from build123d import *

# Parameters (mm, degrees)
SKETCH1_W           = 10.414
SKETCH1_H           = 16.256
BOSS_EXTRUDE1_DEPTH = 3.175
SKETCH2_R           = 1.5875
CUT_EXTRUDE1_DEPTH  = 3.175
SKETCH3_W           = 1.3462
SKETCH3_H           = 0.635
BOSS_EXTRUDE2_DEPTH = 12.7
SKETCH4_W           = 0.2921
SKETCH4_H           = 9.398
CUT_EXTRUDE2_DEPTH  = 3.413


with BuildPart() as part:
    # Sketch1 → Boss-Extrude1 (new body)
    with BuildSketch(Plane(origin=(0, 0, 0), x_dir=(1, 0, 0), z_dir=(0, 1, 0))):
        with Locations((5.207, 8.128)):
            Rectangle(SKETCH1_W, SKETCH1_H)
    extrude(amount=BOSS_EXTRUDE1_DEPTH)

    # Sketch2 → Cut-Extrude1 (cut)
    with BuildSketch(Plane(origin=(0, 3.175, 0), x_dir=(1, 0, 0), z_dir=(0, 1, 0))):
        with Locations((5.207, 13.081)):
            Circle(SKETCH2_R)
        with Locations((10.414, 13.081)):
            Circle(SKETCH2_R)
        with Locations((0, 13.081)):
            Circle(SKETCH2_R)
    extrude(amount=-CUT_EXTRUDE1_DEPTH, mode=Mode.SUBTRACT)

    # Sketch3 → Boss-Extrude2 (add)
    with BuildSketch(Plane.XY):
        with Locations((7.747, 2.0955)):
            Rectangle(SKETCH3_W, SKETCH3_H)
        with Locations((2.667, 2.0955)):
            Rectangle(SKETCH3_W, SKETCH3_H)
    extrude(amount=BOSS_EXTRUDE2_DEPTH)

    # Sketch4 → Cut-Extrude2 (cut, through all)
    with BuildSketch(Plane(origin=(0, 2.413, 0), x_dir=(1, 0, 0), z_dir=(0, 1, 0))):
        with Locations((2.13995, -8.001)):
            Rectangle(SKETCH4_W, SKETCH4_H)
        with Locations((3.19405, -8.001)):
            Rectangle(SKETCH4_W, SKETCH4_H)
        with Locations((7.21995, -8.001)):
            Rectangle(SKETCH4_W, SKETCH4_H)
        with Locations((8.27405, -8.001)):
            Rectangle(SKETCH4_W, SKETCH4_H)
    extrude(amount=-CUT_EXTRUDE2_DEPTH, mode=Mode.SUBTRACT)


solid = part.part
Read the model definition and answer for the solid it produces. Units are mm, in the model's axes. A direction names the side the tool comes from. Round coordinates to 2 decimals unless told otherwise and drop trailing zeros. Write each loop counter-clockwise with the first axis right and the second up, starting at its lowest first coordinate (ties: lowest second). Pieces come first, ordered by that corner, then holes. Notation, with made-up numbers: (-33.75, -37.5) - (20.25, -37.5) arc R16 cw to (20.25, -15.5) - close; hole circle Ø2 at (37, 71). An arc over 180 degrees is marked (long way). Use a Markdown table: item, result.
(1) Each of these flat-tipped pins is pushed along its axis until it touches: pin 1 Ø1.1 at (x, z) = (7.5, 5.5) entering from +Y; pin 2 Ø0.7 at (y, z) = (2, 9) entering from -X; pin 3 Ø1.5 at (x, y) = (1.5, 2.5) entering from +Z. Where does it stop, or does it pass through?
Reported:
| item | result |
|---|---|
| pin 1 | y = 2.41 |
| pin 2 | x = 2.29 |
| pin 3 | z = 3.3 |
(2) The part is cut by section C-C (x = 4). Write down the section's boundary in (y, z) (3 decimals), then the cut area to 3 significant figures.
Reported:
| item | result |
|---|---|
| outline | (0, -16.256) - (3.175, -16.256) - (3.175, -14.112) - (0, -14.112) - close; (0, -12.05) - (3.175, -12.05) - (3.175, 0) - (0, 0) - close |
| area | 45.1 mm2 |
(3) The part is cut by section B-B (y = 1.1). Write down the section's boundary in (x, z) (1 decimal), then the cut area to 3 significant figures.
Reported:
| item | result |
|---|---|
| outline | (0, -16.3) - (10.4, -16.3) - (10.4, -14.7) arc R1.6 cw to (10.4, -11.5) - (10.4, 0) - (0, 0) - (0, -11.5) arc R1.6 cw to (0, -14.7) - close; hole circle Ø3.2 at (5.2, -13.1) |
| area | 153 mm2 |
(4) Straight lines are drawn through the part: line 1 along Z through (x, y) = (7, 1.65); line 2 along X through (y, z) = (1.2, -11.75); line 3 along Z through (x, y) = (0.5, 2.6). For each, find the intervals that lie inside material, in ascending order. Write a range as [from, to].
Reported:
| item | result |
|---|---|
| line 1 | [-16.26, 0] |
| line 2 | [0.87, 4.34], [6.07, 9.55] |
| line 3 | [-16.26, -14.59], [-11.57, 0] |
(5) The part is cut by section A-A (z = 10.25). Write down the section's boundary in (x, y).
Reported:
| item | result |
|---|---|
| outline | (2.29, 1.78) - (3.05, 1.78) - (3.05, 2.41) - (2.29, 2.41) - close; (7.37, 1.78) - (8.13, 1.78) - (8.13, 2.41) - (7.37, 2.41) - close |
(6) The part is cut by section D-D (x = 2.75). Write down the section's boundary in (y, z) (3 decimals).
Reported:
| item | result |
|---|---|
| outline | (0, -16.256) - (3.175, -16.256) - (3.175, 0) - (2.413, 0) - (2.413, 12.7) - (1.778, 12.7) - (1.778, 0) - (0, 0) - close |
(7) Which of the six approach directions +Z, -Z, +X, -X, +Y, -Y give full straight-line access (tool end or side, diameter ignored) to faces 4 (the flat face through (0, 2, -15)), 5 (the flat face through (2.7, 1.778, 4.8)), 6 (the flat face through (7.7, 2.413, 4.8))?
Reported:
| item | result |
|---|---|
| face 4 | +Z, -Z, -X, +Y, -Y |
| face 5 | +Z, +X, -X, -Y |
| face 6 | +Z, +X, -X, +Y |
(8) The mould has two halves that part along Z. Classify faces 1 (the cylindrical face through (8.827, 1.61, -13.116)), 2 (the flat face through (10.414, 2, -15)), 3 (the flat face through (5, 2, -16.256)): released by +Z, released by -Z, zero draft, split by the parting line, or undercut.
Reported:
| item | result |
|---|---|
| face 1 | undercut |
| face 2 | zero draft |
| face 3 | released by -Z |
